Part print with two shaded views. Sizes in mm from the minimum x, y, z corner. A direction names the side the tool comes from. Coordinates: 2 decimals unless noted, no trailing zeros. Write each loop counter-clockwise with the first axis right and the second up, starting at its lowest first coordinate (ties: lowest second). Pieces come first, ordered by that corner, then holes. Notation, with made-up numbers: M -3,8 L 5,8 A26 ccw 5,26 Z; hole C 1.25,9 d10. An arc over 180 degrees is marked long. One line per question, with ' | ' between items. Start each with the question number.
(1) Flat gauge pin, fed straight in: pin 1 Ø6 at (y, z) = (10.5, 12.5) entering from -X. Where does the tip first touch, or does it go through?
(2) Tool access for the marked faces 1 and 2: list every direction of +Z, -Z, +X, -X, +Y, -Y with a clear straight run to the whole face (end or side of a thin tool).
(3) Cut at B-B (y = 12.5). Write the cut outline in (x, z).
(4) Two-plate mould, pull along Z, no slides. Class the marked faces 3, 4 and 5: +Z half, -Z half, draft (parallel to the pull), parting line (faces both ways), or undercut.
(5) Wall check: probe 1 along Z at (x, y) = (16.25, 1); probe 2 along X at (y, z) = (9, 5). Give the ranges that are in metal, low to high.
(6) Cut at A-A (x = 12). Write the cut outline in (y, z).
(7) Cut at C-C (z = 21.5). Write the cut outline in (x, y).
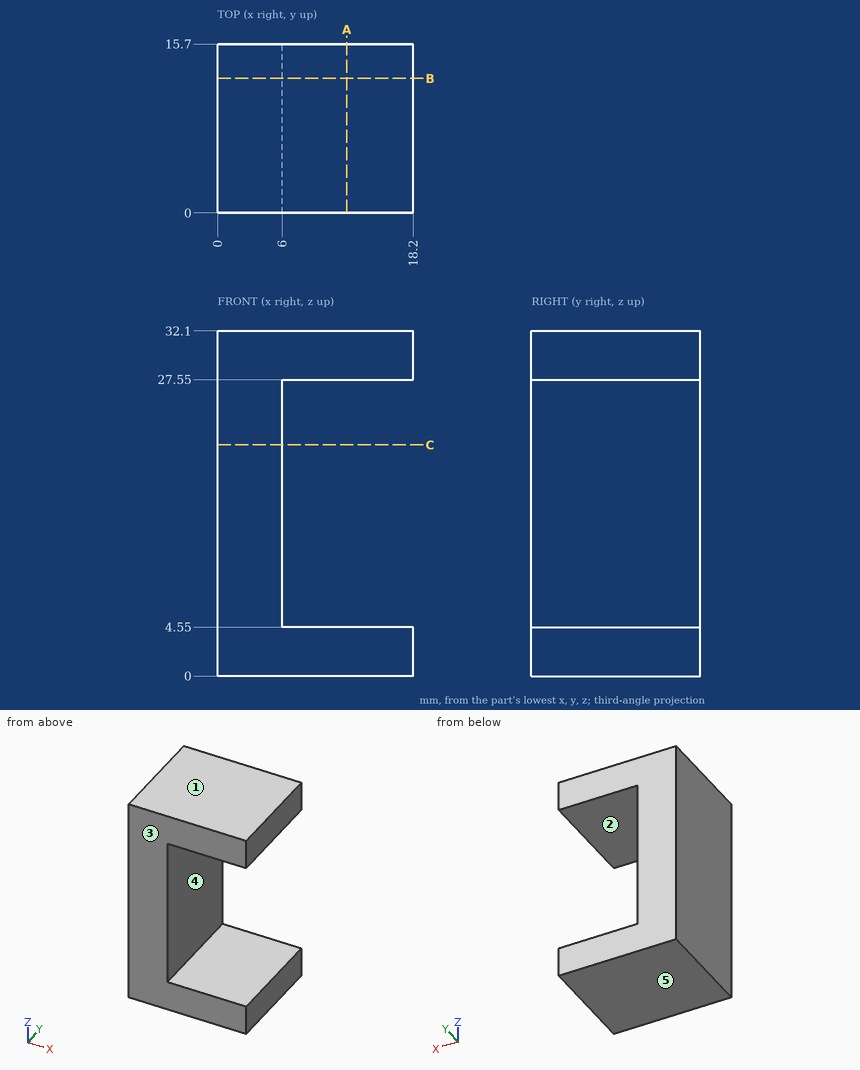
Filled in:
1) pin 1: x = 0
2) face 1: +Z, +X, -X, +Y, -Y | face 2: +X, +Y, -Y
3) outline: M 0,0 L 18.2,0 L 18.2,4.55 L 6,4.55 L 6,27.55 L 18.2,27.55 L 18.2,32.1 L 0,32.1 Z
4) face 3: draft | face 4: undercut | face 5: -Z half
5) probe 1: 0 to 4.55, 27.55 to 32.1 | probe 2: 0 to 6
6) outline: M 0,0 L 15.7,0 L 15.7,4.55 L 0,4.55 Z; M 0,27.55 L 15.7,27.55 L 15.7,32.1 L 0,32.1 Z
7) outline: M 0,0 L 6,0 L 6,15.7 L 0,15.7 Z
